For this review, take the finished solid that the model builds, in its own axes (mm). A direction names the side the tool comes from. Coordinates: 2 decimals unless noted, no trailing zeros. Write each loop counter-clockwise with the first axis right and the second up, starting at its lowest first coordinate (ties: lowest second). Pieces come first, ordered by that corner, then holes.
1) To check wall thickness, follow line 1 along X through (y, z) = (-1.75, -3.5); line 2 along X through (y, z) = (5.25, -7.5); line 3 along Y through (x, z) = (1.25, -1). State the ranges of each line that lie inside material, in increasing order.
2) We need section C-C on x = 4.25. Write out the cut boundary in (y, z).
3) We need section D-D on y = 0.5. Write out the cut boundary in (x, z).
4) Insertion check: P1, Ø0.5, axis at x = -0.5, y = 4, coming from the +Z side; P2, Ø0.5, axis at x = -0.5, y = 6, coming from the -Z side; P3, Ø1, axis at y = 6.5, z = -1, coming from the +X side. Each pin has a flat end and moves straight along its axis. Give the tip position at first contact, or say it passes through.
5) We need section B-B on z = -4.25. Write out the cut boundary in (x, y), then the cut area to 3 significant figures.
6) For faces 1 (the face through (1, 10.5, -4)), 2 (the face through (6.75, -3, -4)), 3 (the face through (13, 4, -1)), 4 (the face through (13.5, 4.4, -6.5)), list the 3-axis set-ups (+Z, -Z, +X, -X, +Y, -Y) from which the entire face can be reached by the end or side of a thin tool; tool diameter is ignored.
7) We need section A-A on y = -3.75. Write out the cut boundary in (x, z), then the cut area to 3 significant figures.
from build123d import *

# Parameters (mm, degrees)
ESQUISSE1_W        = 13
ESQUISSE1_H        = 8.5
ESQUISSE1_W_2      = 1
ESQUISSE1_H_2      = 4.5
BOSS_EXTRU_1_DEPTH = 9
ESQUISSE2_W        = 15
ESQUISSE2_H        = 10.5
BOSS_EXTRU_2_DEPTH = 1.5
CONG_1_R           = 1
ESQUISSE3_W        = 0.5
ESQUISSE3_H        = 3.6
BOSS_EXTRU_3_DEPTH = 6.5
BOSS_EXTRU_4_DEPTH = 8.5


with BuildPart() as part:
    # Esquisse1 → Boss.-Extru.1 (new body)
    with BuildSketch(Plane(origin=(0, 0, 0), x_dir=(1, 0, 0), z_dir=(0, 1, 0))):
        with Locations((6.5, 4.25)):
            Rectangle(ESQUISSE1_W, ESQUISSE1_H)
        with Locations((-0.5, 4.25)):
            Rectangle(ESQUISSE1_W_2, ESQUISSE1_H_2)
        with Locations((13.5, 4.25)):
            Rectangle(ESQUISSE1_W_2, ESQUISSE1_H_2)
    extrude(amount=BOSS_EXTRU_1_DEPTH)

    # Esquisse2 → Boss.-Extru.2 (add)
    with BuildSketch(Plane(origin=(0, 9, 0), x_dir=(1, 0, 0), z_dir=(0, 1, 0))):
        with Locations((6.5, 4.25)):
            Rectangle(ESQUISSE2_W, ESQUISSE2_H)
    extrude(amount=BOSS_EXTRU_2_DEPTH)

    # Congé1
    cong_1_edges = [part.edges().sort_by_distance(p)[0] for p in [
        (-1, 10.5, -4.25),
        (6.5, 10.5, 1),
        (14, 10.5, -4.25),
        (6.5, 10.5, -9.5),
    ]]
    fillet(cong_1_edges, radius=CONG_1_R)

    # Esquisse3 → Boss.-Extru.3 (add)
    with BuildSketch(Plane.XZ):
        with Locations((6.5, -4.25)):
            Rectangle(ESQUISSE3_W, ESQUISSE3_H)
        with Locations((1.5, -4.25)):
            Rectangle(ESQUISSE3_W, ESQUISSE3_H)
        with Locations((11.5, -4.25)):
            Rectangle(ESQUISSE3_W, ESQUISSE3_H)
    extrude(amount=BOSS_EXTRU_3_DEPTH)

    # Esquisse4 → Boss.-Extru.4 (add)
    with BuildSketch(Plane(origin=(0, 0, -8.5), x_dir=(-1, 0, 0), z_dir=(0, 0, -1))):
        with BuildLine():
            ThreePointArc((-11.358192951, 13), (-12.404531, 11.898047996), (-13, 10.5))
            Line((-13, 10.5), (-4.652568423, 10.5))
            Line((-4.652568423, 10.5), (-1.388259271, 10.5))
            ThreePointArc((-1.388259271, 10.5), (-3.07180416, 10.608445517), (-4.743510251, 10.835343224))
            ThreePointArc((-4.743510251, 10.835343224), (-8.130042008, 11.675684327), (-11.358192951, 13))
        make_face()
    extrude(amount=-BOSS_EXTRU_4_DEPTH)


solid = part.part
Result:
1. line 1: x = 1.25 to 1.75, 6.25 to 6.75, 11.25 to 11.75
1. line 2: x = 0 to 13
1. line 3: y = 0 to 10.5
2. outline: (0, -8.5) - (9, -8.5) - (9, -9.5) - (9.5, -9.5) arc R1 ccw to (10.5, -8.5) - (10.76, -8.5) - (10.76, 0) - (10.5, 0) arc R1 ccw to (9.5, 1) - (9, 1) - (9, 0) - (0, 0) - close
3. outline: (-1, -6.5) - (0, -6.5) - (0, -8.5) - (13, -8.5) - (13, -6.5) - (14, -6.5) - (14, -2) - (13, -2) - (13, 0) - (0, 0) - (0, -2) - (-1, -2) - close
4. P1: stops at z = -2
4. P2: stops at z = -6.5
4. P3: stops at x = 13
5. outline: (-1, 0) - (1.25, 0) - (1.25, -6.5) - (1.75, -6.5) - (1.75, 0) - (6.25, 0) - (6.25, -6.5) - (6.75, -6.5) - (6.75, 0) - (11.25, 0) - (11.25, -6.5) - (11.75, -6.5) - (11.75, 0) - (14, 0) - (14, 9.5) arc R1 ccw to (13, 10.5) arc R4.28 ccw to (11.36, 13) arc R23.91 cw to (1.39, 10.5) - (0, 10.5) arc R1 ccw to (-1, 9.5) - close
5. area: 178 mm2
6. face 1: +Z, -Z, -X, +Y
6. face 2: +Z, -Z, -Y
6. face 3: +Z, +X, -Y
6. face 4: -Z, +X, -Y
7. outline: (1.25, -6.05) - (1.75, -6.05) - (1.75, -2.45) - (1.25, -2.45) - close; (6.25, -6.05) - (6.75, -6.05) - (6.75, -2.45) - (6.25, -2.45) - close; (11.25, -6.05) - (11.75, -6.05) - (11.75, -2.45) - (11.25, -2.45) - close
7. area: 5.40 mm2
